Could you check a few things on this drawing? It's one solid part, dimensions in mm from its lowest x, y, z. Round coordinates to 2 decimals unless told otherwise and drop trailing zeros. Order: outer loops, then holes, each group sorted by start corner. A loop starts at its lowest first (then second) coordinate and runs counter-clockwise, first axis right, second up.
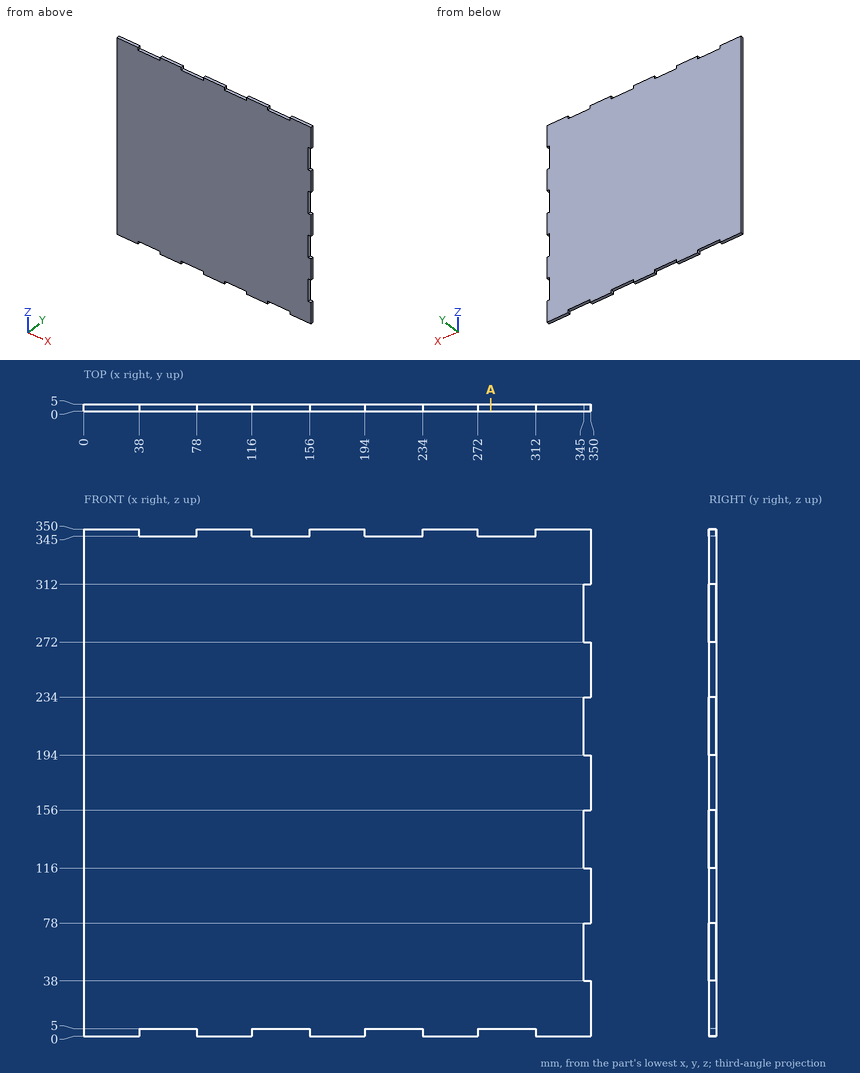
1) If we section it at A-A (x = 281): Write out the boundary of the cut face in (y, z).
2) I need wall thicknesses on line 1 (X direction, y = 4.55, z = 146.5); line 2 (Z direction, x = 289, y = 1). Which ranges of each line are inside material? Lowest first, please.
3) I'm going to push flat-ended pins straight in: pin 1 (1.5 mm diameter, centred on x = 227, y = 2.5, fed in from -Z); pin 2 (3 mm diameter, centred on x = 49.5, y = 1, fed in from +Z); pin 3 (1.5 mm diameter, centred on y = 3, z = 282.5, fed in from +X). Where does each tip first touch, or does it pass through?
Solutions:
1. outline: (0, 5) - (5, 5) - (5, 345) - (0, 345) - close
2. line 1: x = 0 to 345
2. line 2: z = 5 to 345
3. pin 1: stops at z = 5
3. pin 2: stops at z = 345
3. pin 3: stops at x = 345
